Geometry check sheet. Reference: drawing and pictorial views, mm from the part's lowest x, y, z. A direction names the side the tool comes from. Give positions to 0.01 mm unless a question says otherwise; leave off trailing zeros. Loops run counter-clockwise (first coordinate to the right, second up) from the corner with the lowest first, then second, coordinate; pieces in that order, holes last. Notation, with made-up numbers: M -6.75,1 L 21.25,1 A21 cw 21.25,21 Z; hole C 70,54.5 d4. An arc over 180 degrees is marked long. Put each result on its own line as item: value. Start each with the question number.
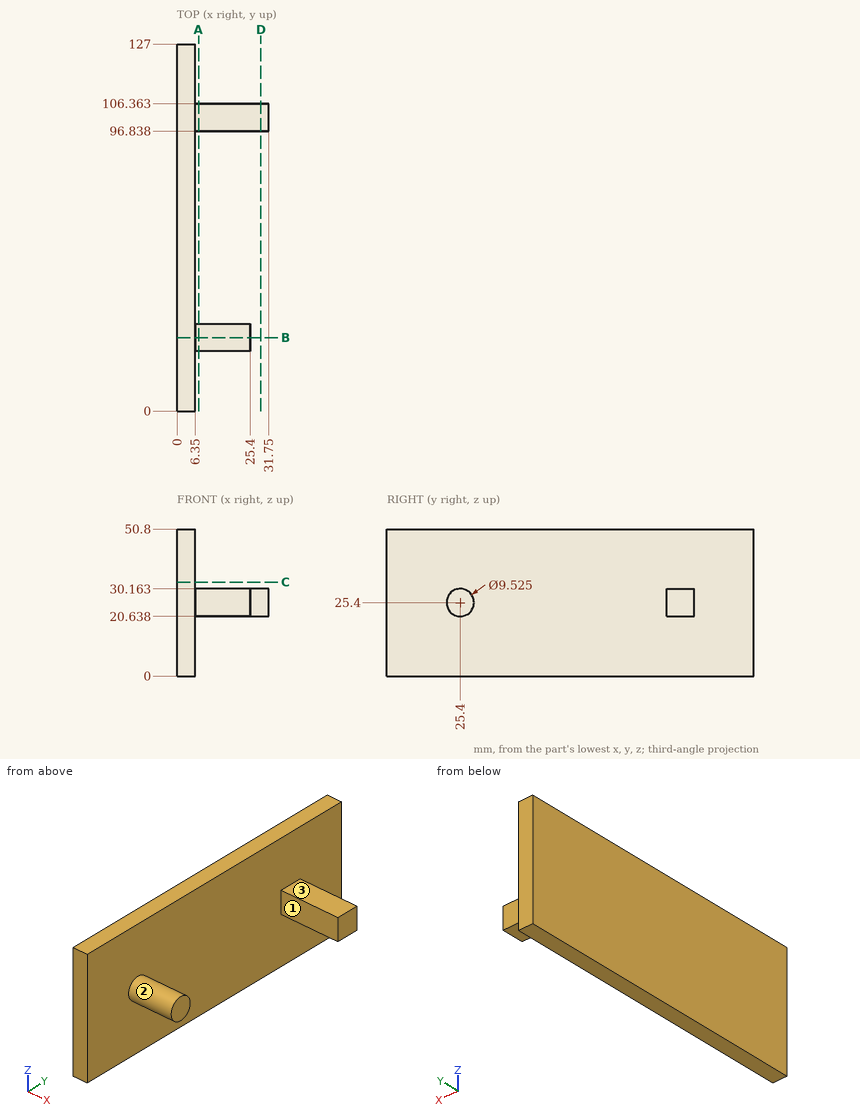
Q1. Access from +Z, -Z, +X, -X, +Y, -Y to the whole of each face (thin tool, end or side, straight path). Record for the marked faces 1, 2 and 3.
Q2. Section check A-A, the plane x = 7.5. Record the cut outline in (y, z) (1 decimal), then the cut area to 3 significant figures.
Q3. Section check D-D, the plane x = 29. Record the cut outline in (y, z).
Q4. Section check B-B, the plane y = 25.4. Record the cut outline in (x, z), then the cut area to 3 significant figures.
Q5. Section check C-C, the plane z = 32.5. Record the cut outline in (x, y).
Q6. Depth check by flat-ended pin: P1, Ø5, axis at x = 24, z = 27, coming from the -Y side; P2, Ø8, axis at x = 22.5, y = 98.5, coming from the +Z side; P3, Ø1.5, axis at y = 66, z = 37.5, coming from the +X side. Enter the tip coordinate at first touch or a pass-through.
Q7. Thickness scan on line 1 along Y through (x, z) = (29.5, 22.5); line 2 along X through (y, z) = (113, 34); line 3 along Y through (x, z) = (18, 26.5) (1 decimal). Record the ranges inside material, lowest first. Write a range as [from, to].
Found:
1. face 1: +Z, -Z, +X
1. face 2: +X
1. face 3: +Z, +X, +Y, -Y
2. outline: C 25.4,25.4 d9.5; M 96.8,20.6 L 106.4,20.6 L 106.4,30.2 L 96.8,30.2 Z
2. area: 162 mm^2
3. outline: M 96.84,20.64 L 106.36,20.64 L 106.36,30.16 L 96.84,30.16 Z
4. outline: M 0,0 L 6.35,0 L 6.35,20.64 L 25.4,20.64 L 25.4,30.16 L 6.35,30.16 L 6.35,50.8 L 0,50.8 Z
4. area: 504 mm^2
5. outline: M 0,0 L 6.35,0 L 6.35,127 L 0,127 Z
6. P1: stops at y = 20.64
6. P2: stops at z = 30.16
6. P3: stops at x = 6.35
7. line 1: y = [96.84, 106.36]
7. line 2: x = [0, 6.35]
7. line 3: y = [20.8, 30], [96.8, 106.4]
